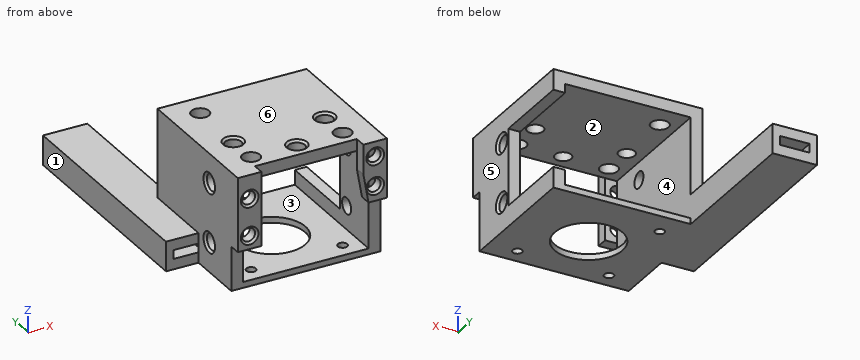
```python
from build123d import *

# Parameters (mm, degrees)
SKETCH2_W                = 50.5
SKETCH2_H                = 40
SKETCH2_W_2              = 42.5
SKETCH2_H_2              = 34
BOSS_EXTRUDE1_DEPTH      = 45
CUT_EXTRUDE1_REACH       = 72.825
SKETCH3_W                = 26
SKETCH3_H                = 27.5
CUT_EXTRUDE2_REACH       = 67.288
SKETCH4_R                = 11.5
SKETCH4_R_2              = 1.6
CUT_EXTRUDE3_REACH       = 67.288
SKETCH5_R                = 3
CUT_EXTRUDE4_REACH       = 67.288
SKETCH6_R                = 2.75
SKETCH7_R                = 2.75
CUT_EXTRUDE5_DEPTH       = 71.825489762
SKETCH8_W                = 8
SKETCH8_H                = 25
BOSS_EXTRUDE2_DEPTH      = 4
SKETCH9_R                = 2.25
CUT_EXTRUDE6_DEPTH       = 4
CHAMFER1_SIZE            = 0.75
BOSS_EXTRUDE3_DEPTH      = 50
BOSS_EXTRUDE3_DEPTH_BACK = 25
SKETCH10_W               = 15
SKETCH10_H               = 10
SKETCH11_W               = 10
SKETCH11_H               = 3
CUT_EXTRUDE7_DEPTH       = 75


with BuildPart() as part:
    # Sketch2 → Boss-Extrude1 (new body)
    with BuildSketch(Plane(origin=(0, 0, 0), x_dir=(1, 0, 0), z_dir=(0, 1, 0))):
        with Locations((0, -1)):
            Rectangle(SKETCH2_W, SKETCH2_H)
        Rectangle(SKETCH2_W_2, SKETCH2_H_2, mode=Mode.SUBTRACT)
    extrude(amount=BOSS_EXTRUDE1_DEPTH)

    # Sketch3 → Cut-Extrude1 (cut, up to next)
    with BuildSketch(Plane(origin=(25.25, 0, 0), x_dir=(0, 0, -1), z_dir=(1, 0, 0)), mode=Mode.PRIVATE) as cut_extrude1_sk1:
        with Locations((-1, 31.25)):
            Rectangle(SKETCH3_W, SKETCH3_H)
    cut_extrude1_tool1 = extrude(cut_extrude1_sk1.sketch, amount=-CUT_EXTRUDE1_REACH, mode=Mode.PRIVATE) & part.part
    add(cut_extrude1_tool1.solids().sort_by_distance((25.25, 31.25, 1))[0], mode=Mode.SUBTRACT)

    # Sketch4 → Cut-Extrude2 (cut, up to next)
    with BuildSketch(Plane(origin=(0, 0, -19), x_dir=(-1, 0, 0), z_dir=(0, 0, -1)), mode=Mode.PRIVATE) as cut_extrude2_sk1:
        with Locations((0, 21)):
            Circle(SKETCH4_R)
    cut_extrude2_tool1 = extrude(cut_extrude2_sk1.sketch, amount=-CUT_EXTRUDE2_REACH, mode=Mode.PRIVATE) & part.part
    # Sketch4 → Cut-Extrude2 (cut, up to next)
    with BuildSketch(Plane(origin=(0, 0, -19), x_dir=(-1, 0, 0), z_dir=(0, 0, -1)), mode=Mode.PRIVATE) as cut_extrude2_sk2:
        with Locations((-15.5, 5.5)):
            Circle(SKETCH4_R_2)
    cut_extrude2_tool2 = extrude(cut_extrude2_sk2.sketch, amount=-CUT_EXTRUDE2_REACH, mode=Mode.PRIVATE) & part.part
    # Sketch4 → Cut-Extrude2 (cut, up to next)
    with BuildSketch(Plane(origin=(0, 0, -19), x_dir=(-1, 0, 0), z_dir=(0, 0, -1)), mode=Mode.PRIVATE) as cut_extrude2_sk3:
        with Locations((15.5, 5.5)):
            Circle(SKETCH4_R_2)
    cut_extrude2_tool3 = extrude(cut_extrude2_sk3.sketch, amount=-CUT_EXTRUDE2_REACH, mode=Mode.PRIVATE) & part.part
    # Sketch4 → Cut-Extrude2 (cut, up to next)
    with BuildSketch(Plane(origin=(0, 0, -19), x_dir=(-1, 0, 0), z_dir=(0, 0, -1)), mode=Mode.PRIVATE) as cut_extrude2_sk4:
        with Locations((15.5, 36.5)):
            Circle(SKETCH4_R_2)
    cut_extrude2_tool4 = extrude(cut_extrude2_sk4.sketch, amount=-CUT_EXTRUDE2_REACH, mode=Mode.PRIVATE) & part.part
    add(cut_extrude2_tool1.solids().sort_by_distance((0, 21, -19))[0], mode=Mode.SUBTRACT)
    add(cut_extrude2_tool2.solids().sort_by_distance((15.5, 5.5, -19))[0], mode=Mode.SUBTRACT)
    add(cut_extrude2_tool3.solids().sort_by_distance((-15.5, 5.5, -19))[0], mode=Mode.SUBTRACT)
    add(cut_extrude2_tool4.solids().sort_by_distance((-15.5, 36.5, -19))[0], mode=Mode.SUBTRACT)

    # Sketch5 → Cut-Extrude3 (cut, up to next)
    with BuildSketch(Plane.XY.offset(21), mode=Mode.PRIVATE) as cut_extrude3_sk1:
        with Locations((-15.5, 36.5)):
            Circle(SKETCH5_R)
    cut_extrude3_tool1 = extrude(cut_extrude3_sk1.sketch, amount=-CUT_EXTRUDE3_REACH, mode=Mode.PRIVATE) & part.part
    # Sketch5 → Cut-Extrude3 (cut, up to next)
    with BuildSketch(Plane.XY.offset(21), mode=Mode.PRIVATE) as cut_extrude3_sk2:
        with Locations((-15.5, 5.5)):
            Circle(SKETCH5_R)
    cut_extrude3_tool2 = extrude(cut_extrude3_sk2.sketch, amount=-CUT_EXTRUDE3_REACH, mode=Mode.PRIVATE) & part.part
    # Sketch5 → Cut-Extrude3 (cut, up to next)
    with BuildSketch(Plane.XY.offset(21), mode=Mode.PRIVATE) as cut_extrude3_sk3:
        with Locations((15.5, 5.5)):
            Circle(SKETCH5_R)
    cut_extrude3_tool3 = extrude(cut_extrude3_sk3.sketch, amount=-CUT_EXTRUDE3_REACH, mode=Mode.PRIVATE) & part.part
    add(cut_extrude3_tool1.solids().sort_by_distance((-15.5, 36.5, 21))[0], mode=Mode.SUBTRACT)
    add(cut_extrude3_tool2.solids().sort_by_distance((-15.5, 5.5, 21))[0], mode=Mode.SUBTRACT)
    add(cut_extrude3_tool3.solids().sort_by_distance((15.5, 5.5, 21))[0], mode=Mode.SUBTRACT)

    # Sketch6 → Cut-Extrude4 (cut, up to next)
    with BuildSketch(Plane.XY.offset(21), mode=Mode.PRIVATE) as cut_extrude4_sk1:
        with Locations((-15.5, 16.365063509)):
            Circle(SKETCH6_R)
    cut_extrude4_tool1 = extrude(cut_extrude4_sk1.sketch, amount=-CUT_EXTRUDE4_REACH, mode=Mode.PRIVATE) & part.part
    # Sketch6 → Cut-Extrude4 (cut, up to next)
    with BuildSketch(Plane.XY.offset(21), mode=Mode.PRIVATE) as cut_extrude4_sk2:
        with Locations((0, 5.5)):
            Circle(SKETCH6_R)
    cut_extrude4_tool2 = extrude(cut_extrude4_sk2.sketch, amount=-CUT_EXTRUDE4_REACH, mode=Mode.PRIVATE) & part.part
    # Sketch6 → Cut-Extrude4 (cut, up to next)
    with BuildSketch(Plane.XY.offset(21), mode=Mode.PRIVATE) as cut_extrude4_sk3:
        with Locations((15.5, 16.365063509)):
            Circle(SKETCH6_R)
    cut_extrude4_tool3 = extrude(cut_extrude4_sk3.sketch, amount=-CUT_EXTRUDE4_REACH, mode=Mode.PRIVATE) & part.part
    add(cut_extrude4_tool1.solids().sort_by_distance((-15.5, 16.365064, 21))[0], mode=Mode.SUBTRACT)
    add(cut_extrude4_tool2.solids().sort_by_distance((0, 5.5, 21))[0], mode=Mode.SUBTRACT)
    add(cut_extrude4_tool3.solids().sort_by_distance((15.5, 16.365064, 21))[0], mode=Mode.SUBTRACT)

    # Sketch7 → Cut-Extrude5 (cut, through all)
    with BuildSketch(Plane(origin=(25.25, 0, 0), x_dir=(0, 0, -1), z_dir=(1, 0, 0))):
        with Locations((-11, 13.440603491)):
            Circle(SKETCH7_R)
        with Locations((9, 13.440603491)):
            Circle(SKETCH7_R)
    extrude(amount=-CUT_EXTRUDE5_DEPTH, mode=Mode.SUBTRACT)

    # Sketch8 → Boss-Extrude2 (add)
    with BuildSketch(Plane.XZ):
        Polygon((19, 1), (17.25, 11), (17.25, 21), (25.25, 21), (25.25, 1), align=None)
        with Locations((-21.25, 8.5)):
            Rectangle(SKETCH8_W, SKETCH8_H)
    extrude(amount=BOSS_EXTRUDE2_DEPTH)

    # Sketch9 → Cut-Extrude6 (cut)
    with BuildSketch(Plane.XZ.offset(4)):
        with Locations(Location((-21.25, 13, 0), (0, 0, 270))):
            Circle(SKETCH9_R)
        with Locations(Location((-21.25, 0.5, 0), (0, 0, 270))):
            Circle(SKETCH9_R)
        with Locations(Location((21.25, 6, 0), (0, 0, 270))):
            Circle(SKETCH9_R)
        with Locations(Location((21.25, 16, 0), (0, 0, 270))):
            Circle(SKETCH9_R)
    extrude(amount=-CUT_EXTRUDE6_DEPTH, mode=Mode.SUBTRACT)

    # Chamfer1
    chamfer1_edges = [part.edges().sort_by_distance(p)[0] for p in [
        (21.25, -4, 18.25),
        (21.25, -4, 8.25),
        (-21.25, -4, 2.75),
        (-21.25, -4, 15.25),
        (-18.25, 16.365063509, 21),
        (-2.75, 5.5, 21),
        (12.75, 16.365063509, 21),
        (-25.25, 13.440603491, 13.75),
        (25.25, 13.440603491, 13.75),
        (-25.25, 13.440603491, -6.25),
        (25.25, 13.440603491, -6.25),
    ]]
    chamfer(chamfer1_edges, length=CHAMFER1_SIZE)

    # Sketch10 → Boss-Extrude3 (add, two sides: drawn at the far end of the back side and taken through both)
    with BuildSketch(Plane(origin=(0, 45, 0), x_dir=(1, 0, 0), z_dir=(0, 1, 0)).offset(-BOSS_EXTRUDE3_DEPTH_BACK)):
        with Locations((-28.75, 14)):
            Rectangle(SKETCH10_W, SKETCH10_H)
    extrude(amount=BOSS_EXTRUDE3_DEPTH + BOSS_EXTRUDE3_DEPTH_BACK)

    # Sketch11 → Cut-Extrude7 (cut)
    with BuildSketch(Plane(origin=(0, 95, 0), x_dir=(1, 0, 0), z_dir=(0, 1, 0))):
        with Locations((-28.75, 14)):
            Rectangle(SKETCH11_W, SKETCH11_H)
    extrude(amount=-CUT_EXTRUDE7_DEPTH, mode=Mode.SUBTRACT)


solid = part.part
```
Here's how the part is built. I have some questions about the finished solid (model axes, mm). Face numbers are marked on the shaded views. A direction names the side the tool comes from. Round coordinates to 2 decimals unless told otherwise and drop trailing zeros. Loops run counter-clockwise (first coordinate to the right, second up) from the corner with the lowest first, then second, coordinate; pieces in that order, holes last.
1. Will these pins go through, and if not, where does the flat tip stop? pin 1 (1.8 mm diameter, centred on x = 22, z = 5.5, fed in from -Y); pin 2 (4.5 mm diameter, centred on x = -30, y = 53, fed in from +Z); pin 3 (2 mm diameter, centred on x = -7.5, z = -17, fed in from +Y); pin 4 (12 mm diameter, centred on x = 5, y = 24.5, fed in from -Z).
Answers:
pin 1: stops at y = 0
pin 2: stops at z = -9
pin 3: stops at y = 45
pin 4: stops at z = -19
2. Suppose I cut it at C-C, the plane y = 23. Please give me the cut outline in (x, z), and give its area (3 significant figures).
Answers:
outline: (-36.25, -19) - (-11.32, -19) - (-11.32, -17) - (-21.25, -17) - (-21.25, 17) - (21.25, 17) - (21.25, 14) - (25.25, 14) - (25.25, 21) - (-25.25, 21) - (-25.25, -9) - (-36.25, -9) - close; (11.32, -19) - (25.25, -19) - (25.25, -12) - (21.25, -12) - (21.25, -17) - (11.32, -17) - close; hole (-33.75, -15.5) - (-23.75, -15.5) - (-23.75, -12.5) - (-33.75, -12.5) - close
area: 506 mm2
3. Suppose I cut it at A-A, the plane y = 36.5. Please give me the cut outline in (x, z), and give its area (3 significant figures).
Answers:
outline: (-36.25, -19) - (-17.1, -19) - (-17.1, -17) - (-21.25, -17) - (-21.25, 17) - (-18.5, 17) - (-18.5, 21) - (-25.25, 21) - (-25.25, -9) - (-36.25, -9) - close; (-13.9, -19) - (25.25, -19) - (25.25, -12) - (21.25, -12) - (21.25, -17) - (-13.9, -17) - close; (-12.5, 17) - (21.25, 17) - (21.25, 14) - (25.25, 14) - (25.25, 21) - (-12.5, 21) - close; hole (-33.75, -15.5) - (-23.75, -15.5) - (-23.75, -12.5) - (-33.75, -12.5) - close
area: 521 mm2
4. For the marked faces 1, 2 and 3, which set-ups out of +Z, -Z, +X, -X, +Y, -Y let a thin tool reach every point of the face, with its end or its side?
Answers:
face 1: +Z, -Z, -X, +Y, -Y
face 2: +Y
face 3: +Y, -Y
5. Suppose I cut it at D-D, the plane x = -15.5. Give the number of separate pieces and of enclosed holes in the cut face, and give its area (3 significant figures).
Answers:
separate pieces: 7
enclosed holes: 0
area: 187 mm2
6. Thinking about a two-plate mould opening in Z: for the marked faces 4, 5 and 6, which applies, released by +Z, released by -Z, zero draft, split by the parting line, or undercut?
Answers:
face 4: undercut
face 5: zero draft
face 6: released by +Z
7. Suppose I cut it at B-B, the plane x = 15.5. Please give me the cut outline in (y, z), and give its area (3 significant figures).
Answers:
outline: (0, -19) - (3.9, -19) - (3.9, -17) - (0, -17) - close; (0, 17) - (2.5, 17) - (2.5, 21) - (0, 21) - close; (7.1, -19) - (45, -19) - (45, -17) - (7.1, -17) - close; (8.5, 17) - (13.62, 17) - (13.62, 20.25) - (12.87, 21) - (8.5, 21) - close; (19.12, 17) - (45, 17) - (45, 21) - (19.87, 21) - (19.12, 20.25) - close
area: 217 mm2
8. If I drill on probe 1 along X at (y, z) = (-2, 13); probe 2 along Z at (x, y) = (-30.5, 84.5); probe 3 along X at (y, z) = (13, -3), over which ranges is the centre line in solid material (lowest first)?
Answers:
probe 1: x = -25.25 to -23.5, -19 to -17.25, 17.25 to 25.25
probe 2: z = -19 to -15.5, -12.5 to -9
probe 3: x = -25.25 to -21.25, 21.25 to 25.25
